Source: CAD feature listing. Evaluate the final solid. Frame: model axes, mm. Face numbers are marked on the shaded views. A direction names the side the tool comes from. Give positions to 0.01 mm unless a question says otherwise; leave off trailing zeros. Order: outer loops, then holes, each group sorted by start corner. A loop starts at its lowest first (then second) coordinate and runs counter-clockwise, first axis right, second up.
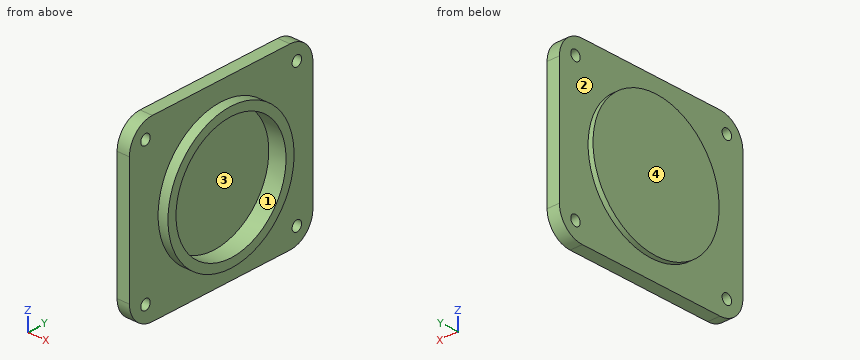
Autodesk Inventor part; units mm, degrees
ref_plane "YZ Plane" through (0, 0, 0) normal (1, 0, 0) x (0, 1, 0)
ref_plane "XZ Plane" through (0, 0, 0) normal (0, 1, 0) x (-1, 0, 0)
ref_plane "XY Plane" through (0, 0, 0) normal (0, 0, 1) x (1, 0, 0)
sketch "Skizze1" plane through (0, 0, 0) normal (1, 0, 0) x (0, 1, 0)
  line L0 (-43, 62) -> (37, 62)
  line L1 (37, 62) -> (37, -8)
  line L2 (37, -8) -> (-43, -8)
  line L3 (-43, -8) -> (-43, 62)
  line L4 (-43, 62) -> (37, -8) construction
  line L5 (37, 62) -> (-43, -8) construction
  point P0 (-3, 27)
  dimension "d3" = 80
  dimension "d4" = 70
extrude "Extrusion1" add sketch "Skizze1" along normal blind 5
sketch "Skizze2" plane through (5, 0, 0) normal (1, 0, 0) x (0, 0, -1)
  circle A0 centre (-27, -3) radius 27.5
  line L0 (8, 37) -> (-62, 37)
  line L1 (-62, 37) -> (-62, -43)
  point P0 (0, 0)
  dimension "d5" = 55
  dimension "d11" = 40
  dimension "d12" = 35
extrude "Extrusion2" add sketch "Skizze2" along normal blind 4
sketch "Skizze3" plane through (9, -3, 27) normal (1, 0, 0) x (0, 0, -1)
  circle A0 centre (0, 0) radius 24
  point P0 (27, 3)
  dimension "d8" = 48
extrude "Extrusion3" cut sketch "Skizze3" against normal through all
fillet "Rundung1" radius 10 4 edges at (2.5, 37, -8) (2.5, 37, 62) (2.5, -43, 62) (2.5, -43, -8)
sketch "Skizze4" plane through (5, 0, 0) normal (1, 0, 0) x (0, 0, -1)
  circle A0 centre (-27, -3) radius 33.55
  line L0 (-2, 37) -> (-52, 37)
  line L1 (-62, 27) -> (-62, -33)
  line L2 (8, -33) -> (8, 27)
  line L3 (-52, -43) -> (-2, -43)
  point P0 (0, 0)
  point P1 (-55, 30)
  point P2 (1, 30)
  point P3 (1, -36)
  point P4 (-55, -36)
  dimension "d14" = 67.1
  dimension "d15" = 7
  dimension "d16" = 7
  dimension "d17" = 7
  dimension "d18" = 7
  dimension "d19" = 7
  dimension "d20" = 7
  dimension "d21" = 7
  dimension "d29" = 7
hole "Bohrung1" at (5, 30, 55) at (5, 30, -1) at (5, -36, -1) at (5, -36, 55) direction (-1, 0, 0) diameter 4.134 end through all
sketch "Skizze5" plane through (0, 0, 0) normal (-1, 0, 0) x (0, 0, 1)
  circle A0 centre (27, -3) radius 24
  circle A1 centre (27, -3) radius 27.5
  circle A2 centre (27, -3) radius 10
  point P0 (0, 0)
  dimension "d30" = 55
  dimension "d39" = 20
extrude "Extrusion5" add sketch "Skizze5" along normal mid plane 4 contours A0 | A1 | A2
properties part number "Deckel Endewelle" material "Aluminium 6061"
1) Material intervals for L1, parallel to Y at x = 3, z = 55; L2, parallel to Z at x = 2.95, y = -36; L3, parallel to Z at x = 1.75, y = -37, sorted ascending.
Report:
L1: y = -42.54 to -38.07, -33.93 to 27.93, 32.07 to 36.54
L2: z = -7.54 to -3.07, 1.07 to 52.93, 57.07 to 61.54
L3: z = -7.17 to -2.81, 0.81 to 53.19, 56.81 to 61.17
2) Section query B-B, the plane y = -3. Return the cut outline in (x, z).
Report:
outline: (-2, -0.5) - (0, -0.5) - (0, -8) - (5, -8) - (5, -0.5) - (9, -0.5) - (9, 3) - (2, 3) - (2, 51) - (9, 51) - (9, 54.5) - (5, 54.5) - (5, 62) - (0, 62) - (0, 54.5) - (-2, 54.5) - close
3) Pin query (flat end, axial travel): pin 1 (5 mm diameter, centred on y = 30, z = -1, fed in from +X); pin 2 (3.5 mm diameter, centred on y = -36, z = 55, fed in from +X). Return the tip coordinate at first contact, or that it passes through.
Report:
pin 1: stops at x = 5
pin 2: passes through
4) Reachability of the marked faces 3 and 4 from +Z, -Z, +X, -X, +Y, -Y: full face, straight path, thin tool, end or side. Return the list, or none.
Report:
face 3: +X
face 4: +Z, -Z, -X, +Y, -Y
5) Section query A-A, the plane x = 3.5. Return the cut outline in (y, z).
Report:
outline: (-43, 2) arc R10 ccw to (-33, -8) - (27, -8) arc R10 ccw to (37, 2) - (37, 52) arc R10 ccw to (27, 62) - (-33, 62) arc R10 ccw to (-43, 52) - close; hole circle Ø4.13 at (-36, -1); hole circle Ø4.13 at (-36, 55); hole circle Ø48 at (-3, 27); hole circle Ø4.13 at (30, -1); hole circle Ø4.13 at (30, 55)
6) Section query C-C, the plane z = 16. Return the cut outline in (x, y), and give its area (3 significant figures).
Report:
outline: (-2, -28.2) - (0, -28.2) - (0, -43) - (5, -43) - (5, -28.2) - (9, -28.2) - (9, -24.33) - (2, -24.33) - (2, 18.33) - (9, 18.33) - (9, 22.2) - (5, 22.2) - (5, 37) - (0, 37) - (0, 22.2) - (-2, 22.2) - close
area: 404 mm2
7) Draft query along Z for the marked faces 1 and 2. Return one class per face: +Z half, -Z half, draft (parallel to the pull), parting line (faces both ways), or undercut.
Report:
face 1: undercut
face 2: draft
8) Section query D-D, the plane y = 30. Return the cut outline in (x, z), and give its area (3 significant figures).
Report:
outline: (0, -7.54) - (5, -7.54) - (5, -3.07) - (0, -3.07) - close; (0, 1.07) - (5, 1.07) - (5, 52.93) - (0, 52.93) - close; (0, 57.07) - (5, 57.07) - (5, 61.54) - (0, 61.54) - close
area: 304 mm2
